Solid Edge part; units mm, degrees
sketch "Sketch1" plane through (0, 0, 0) normal (0, 0, 1) x (1, 0, 0)
  line L0 (-25.4, 15.875) -> (25.4, 15.875)
  line L1 (25.4, 15.875) -> (25.4, 9.525)
  line L2 (25.4, 9.525) -> (9.525, 9.525)
  line L3 (9.525, 9.525) -> (9.525, -9.525)
  line L4 (9.525, -9.525) -> (-9.525, -9.525)
  line L5 (-9.525, -9.525) -> (-9.525, 9.525)
  line L6 (-9.525, 9.525) -> (-25.4, 9.525)
  line L7 (-25.4, 9.525) -> (-25.4, 15.875)
  dimension "D1" = 25.4
  dimension "D2" = 9.525
  dimension "D3" = 25.4
  dimension "D4" = 25.4
  dimension "D5" = 9.525
  dimension "D6" = 25.4
  dimension "D7" = 9.525
  dimension "D8" = 9.525
extrude "Protrusion1" add sketch "Sketch1" along normal blind 12.7
fillet "Round_1" radius 3.175 6 edges at (9.525, 9.525, 6.35) (9.525, -9.525, 6.35) (-9.525, -9.525, 6.35) (25.4, 9.525, 6.35) (-9.525, 9.525, 6.35) (-25.4, 9.525, 6.35)
sketch "Sketch2" plane through (0, 3.175, 12.7) normal (0, 0, 1) x (0, 1, 0)
  circle A0 centre (-3.175, 0) radius 6.35
extrude "PivotHole" cut sketch "Sketch2" against normal blind 10.16
sketch "Sketch3" plane through (-17.4625, 9.525, 6.35) normal (0, -1, 0) x (1, 0, 0)
  circle A0 centre (-0.3175, 0) radius 3.175
  dimension "D1" = 0.3175
extrude "v_1" cut sketch "Sketch3" against normal blind 25.4
mirror "Mirror1" about plane through (0, 0, 0) normal (1, 0, 0) of "v_1"
properties material "Aluminum, 6061-T6"
Check sheet for the modelled part. Datum: model origin and axes. Units: mm. A direction names the side the tool comes from. Give positions to 0.01 mm unless a question says otherwise; leave off trailing zeros. Loops run counter-clockwise (first coordinate to the right, second up) from the corner with the lowest first, then second, coordinate; pieces in that order, holes last. Notation, with made-up numbers: (61.25, 62) - (87.25, 62) arc R12 ccw to (87.25, 72) - close; hole circle Ø2 at (45.25, 20.25). An arc over 180 degrees is marked (long way). One line per question, with ' | ' between items. Start each with the question number.
1. Cross-section at C-C, the plane z = 10.25. Enter the section's corners in (x, y) (3 decimals).
2. Gauge pin test, flat ends, axial feed: pin 1 Ø4 at (x, y) = (-2.5, 0) entering from +Z; pin 2 Ø4 at (x, z) = (17.78, 6.35) entering from -Y (3 decimals); pin 3 Ø6 at (y, z) = (7, 2) entering from -X; pin 4 Ø4 at (y, z) = (0.5, 9.5) entering from -X (3 decimals). Record the tip position at first contact, or that the pin passes through.
3. Cross-section at B-B, the plane z = 6.35. Enter the section's corners in (x, y) (3 decimals).
4. Set-up check for faces 1 (the flat face through (16, 9.525, 3)), 2 (the flat face through (0, 9, 12.7)), 3 (the flat face through (-16, 9.525, 3)): record each of +Z, -Z, +X, -X, +Y, -Y from which the full face is reachable in a straight line by a thin tool's end or side.
5. Cross-section at D-D, the plane y = 0. Enter the section's corners in (x, z) (3 decimals).
6. Draft check along Y on faces 4 (the flat face through (0, 0, 2.54)), 5 (the cylindrical face through (8.57, -8.62, 6.44)), 6 (the flat face through (-25.4, 14, 6)). Enter one of: released by +Y, released by -Y, zero draft, split by the parting line, or undercut.
7. Material ranges on line 1 along Y through (x, z) = (0, 9) (3 decimals); line 2 along X through (y, z) = (-0.25, 2.75) (3 decimals); line 3 along Z through (x, y) = (-18, 11.25), recorded low to high. Write a range as [from, to].
8. Cross-section at A-A, the plane x = -17.78. Enter the section's corners in (y, z) (3 decimals).
Check result:
1) outline: (-25.4, 12.7) arc R3.175 ccw to (-22.225, 9.525) - (-12.7, 9.525) arc R3.175 cw to (-9.525, 6.35) - (-9.525, -6.35) arc R3.175 ccw to (-6.35, -9.525) - (6.35, -9.525) arc R3.175 ccw to (9.525, -6.35) - (9.525, 6.35) arc R3.175 cw to (12.7, 9.525) - (22.225, 9.525) arc R3.175 ccw to (25.4, 12.7) - (25.4, 15.875) - (-25.4, 15.875) - close; hole circle Ø12.7 at (0, 0)
2) pin 1: stops at z = 2.54 | pin 2: passes through | pin 3: stops at x = -23.9 | pin 4: stops at x = -9.525
3) outline: (-25.4, 12.7) arc R3.175 ccw to (-22.225, 9.525) - (-20.955, 9.525) - (-20.955, 15.875) - (-25.4, 15.875) - close; (-14.605, 9.525) - (-12.7, 9.525) arc R3.175 cw to (-9.525, 6.35) - (-9.525, -6.35) arc R3.175 ccw to (-6.35, -9.525) - (6.35, -9.525) arc R3.175 ccw to (9.525, -6.35) - (9.525, 6.35) arc R3.175 cw to (12.7, 9.525) - (14.605, 9.525) - (14.605, 15.875) - (-14.605, 15.875) - close; (20.955, 9.525) - (22.225, 9.525) arc R3.175 ccw to (25.4, 12.7) - (25.4, 15.875) - (20.955, 15.875) - close; hole circle Ø12.7 at (0, 0)
4) face 1: +Z, -Z, +X, -Y | face 2: +Z, +X, -X, +Y, -Y | face 3: +Z, -Z, -X, -Y
5) outline: (-9.525, 0) - (9.525, 0) - (9.525, 12.7) - (6.35, 12.7) - (6.35, 2.54) - (-6.35, 2.54) - (-6.35, 12.7) - (-9.525, 12.7) - close
6) face 4: undercut | face 5: released by -Y | face 6: zero draft
7) line 1: y = [-9.525, -6.35], [6.35, 15.875] | line 2: x = [-9.525, -6.345], [6.345, 9.525] | line 3: z = [0, 3.18], [9.52, 12.7]
8) outline: (9.525, 0) - (15.875, 0) - (15.875, 3.175) - (9.525, 3.175) - close; (9.525, 9.525) - (15.875, 9.525) - (15.875, 12.7) - (9.525, 12.7) - close
